```python
from build123d import *

# Parameters (mm, degrees)
BASE_EXTRUDE_DEPTH = 4.7625
CHAMFER1_SIZE      = 6.35


with BuildPart() as part:
    # Sketch1 → Base-Extrude (new body, symmetric)
    with BuildSketch(Plane(origin=(0, 0, 0), x_dir=(1, 0, 0), z_dir=(0, 1, 0))):
        Polygon((0, 0), (44.45, 0), (44.45, 25.4), (19.05, 44.45), (0, 44.45), align=None)
    extrude(amount=BASE_EXTRUDE_DEPTH, both=True)

    # Chamfer1
    chamfer1_edges = [part.edges().sort_by_distance(p)[0] for p in [
        (0, 0, 0),
    ]]
    chamfer(chamfer1_edges, length=CHAMFER1_SIZE)


solid = part.part
```
Work out the finished part from the listing and answer in its coordinate system (mm). Round coordinates to 2 decimals unless told otherwise and drop trailing zeros. Order: outer loops, then holes, each group sorted by start corner. A loop starts at its lowest first (then second) coordinate and runs counter-clockwise, first axis right, second up.
Q1. A cutting plane is placed at C-C, the plane x = 3. Determine the outline of the cut face in (y, z), then the cut area to 3 significant figures.
Solution:
outline: (-4.76, -44.45) - (4.76, -44.45) - (4.76, -3.35) - (-4.76, -3.35) - close
area: 391 mm2
Q2. A cutting plane is placed at A-A, the plane y = -1.5. Determine the outline of the cut face in (x, z), then the cut area to 3 significant figures.
Solution:
outline: (0, -44.45) - (19.05, -44.45) - (44.45, -25.4) - (44.45, 0) - (6.35, 0) - (0, -6.35) - close
area: 1,710 mm2
Q3. Find the intervals of material crossed by line 1 along Z through (x, y) = (19.5, -2); line 2 along Z through (x, y) = (35, -2); line 3 along X through (y, z) = (-2.5, -2), in increasing order.
Solution:
line 1: z = -44.11 to 0
line 2: z = -32.49 to 0
line 3: x = 4.35 to 44.45
Q4. A cutting plane is placed at B-B, the plane z = -5.5. Determine the outline of the cut face in (x, y).
Solution:
outline: (0.85, -4.76) - (44.45, -4.76) - (44.45, 4.76) - (0.85, 4.76) - close
